Input: part model. Units: mm. Frame: model coordinates. Give positions to 0.01 mm unless a question says otherwise; leave off trailing zeros. Write each loop counter-clockwise with the first axis right and the second up, starting at its lowest first coordinate (ties: lowest second). Pieces come first, ordered by that corner, then holes. Notation, with made-up numbers: (-30, -14) - (23, -14) arc R14 ccw to (23, 6) - close; hole circle Ø7 at (-12, -19). An arc over 180 degrees is marked (long way). Use a Markdown table: item, result. Add a question column.
1. Section query B-B, the plane x = 51. Return loops of the section in (y, z), plus the area to 3 significant figures.
2. Material intervals for probe 1 along Y at (x, z) = (-43.5, -64.5), sorted ascending.
3. Section query C-C, the plane x = 139.5. Return loops of the section in (y, z), plus the area to 4 significant figures.
4. Section query A-A, the plane z = 9.5. Return loops of the section in (x, y), plus the area to 3 significant figures.
5. Pin query (flat end, axial travel): pin 1 (12 mm diameter, centred on x = -58, z = -36.5, fed in from -Y); pin 2 (2 mm diameter, centred on x = 101.5, z = 53.5, fed in from +Y); pin 3 (0.6 mm diameter, centred on y = -0.5, z = 70.5, fed in from +X). Return the tip coordinate at first contact, or that it passes through.
```python
from build123d import *

# Parameters (mm, degrees)
SKETCH1_W           = 350
SKETCH1_H           = 200
SKETCH1_W_2         = 28
SKETCH1_H_2         = 7
BOSS_EXTRUDE3_DEPTH = 6.45
SKETCH1_4_W         = 360
SKETCH1_4_H         = 210
SKETCH1_4_W_2       = 350
SKETCH1_4_H_2       = 200
BOSS_EXTRUDE4_DEPTH = 6.5
SKETCH1_5_W         = 28
SKETCH1_5_H         = 7
BOSS_EXTRUDE5_DEPTH = 0.5


with BuildPart() as part:
    # Sketch1 → Boss-Extrude3 (new body)
    with BuildSketch(Plane(origin=(0, 0, 0), x_dir=(1, 0, 0), z_dir=(0, 1, 0))):
        Rectangle(SKETCH1_W, SKETCH1_H)
        with Locations((61, -68.9)):
            Rectangle(SKETCH1_W_2, SKETCH1_H_2, mode=Mode.SUBTRACT)
        with Locations((61, -68.9)):
            Rectangle(SKETCH1_W_2, SKETCH1_H_2)
    extrude(amount=BOSS_EXTRUDE3_DEPTH)

    # Sketch1_4 → Boss-Extrude4 (add)
    with BuildSketch(Plane(origin=(0, 0, 0), x_dir=(1, 0, 0), z_dir=(0, 1, 0))):
        Rectangle(SKETCH1_4_W, SKETCH1_4_H)
        Rectangle(SKETCH1_4_W_2, SKETCH1_4_H_2, mode=Mode.SUBTRACT)
    extrude(amount=BOSS_EXTRUDE4_DEPTH)

    # Sketch1_5 → Boss-Extrude5 (add)
    with BuildSketch(Plane(origin=(0, 0, 0), x_dir=(1, 0, 0), z_dir=(0, 1, 0))):
        with Locations((61, -68.9)):
            Rectangle(SKETCH1_5_W, SKETCH1_5_H)
    extrude(amount=-BOSS_EXTRUDE5_DEPTH)


solid = part.part
```
Result sheet:
| question | item | result |
|---|---|---|
| 1 | outline | (-0.5, 65.4) - (0, 65.4) - (0, -105) - (6.5, -105) - (6.5, -100) - (6.45, -100) - (6.45, 100) - (6.5, 100) - (6.5, 105) - (0, 105) - (0, 72.4) - (-0.5, 72.4) - close |
| 1 | area | 1,360 mm² |
| 2 | probe 1 | y = 0 to 6.45 |
| 3 | outline | (0, -105) - (6.5, -105) - (6.5, -100) - (6.45, -100) - (6.45, 100) - (6.5, 100) - (6.5, 105) - (0, 105) - close |
| 3 | area | 1,355 mm² |
| 4 | outline | (-180, 0) - (180, 0) - (180, 6.5) - (175, 6.5) - (175, 6.45) - (-175, 6.45) - (-175, 6.5) - (-180, 6.5) - close |
| 4 | area | 2,320 mm² |
| 5 | pin 1 | stops at y = 0 |
| 5 | pin 2 | stops at y = 6.45 |
| 5 | pin 3 | stops at x = 75 |
